For this review, take the finished solid that the model builds, in its own axes (mm). Round coordinates to 2 decimals unless told otherwise and drop trailing zeros. Write each loop counter-clockwise with the first axis right and the second up, starting at its lowest first coordinate (ties: lowest second). Pieces come first, ordered by that corner, then holes. Notation, with made-up numbers: M 15,-15.5 L 58,-15.5 A24 cw 58,15.5 Z; hole C 8.5,27 d6. An arc over 180 degrees is marked long. Use one line per item in the form item = value. Start each with the question number.
Item 1: For P1, Ø4, axis at x = 19, z = -24.5, coming from the -Y side; P2, Ø1.5, axis at x = -39, z = 24.5, coming from the -Y side, all flat-tipped, find the tip position at first contact; note any pin that passes through.
Item 2: Add section A-A (z = 24.5). State the section outline as (x, y) points, and give its area (3 significant figures).
Item 3: Add section B-B (x = -39). State the section outline as (y, z) points.
Item 4: For line 1 (X direction, y = -0.7, z = -24.5); line 2 (Z direction, x = -39, y = -0.4); line 3 (Z direction, x = 20, y = -0.2), list the stretches that pass through material, from the lowest coordinate up. Write a range as [from, to].
from build123d import *

# Parameters (mm, degrees)
SCHIZZO1_R                   = 1.25
ESTRUSIONE_ESTRUSIONE1_DEPTH = 1.3


with BuildPart() as part:
    # Schizzo1 → Estrusione-Estrusione1 (new body)
    with BuildSketch(Plane(origin=(0, 0, 0), x_dir=(1, 0, 0), z_dir=(0, 1, 0))):
        with BuildLine():
            Line((42.5, -25.5), (42.5, 25.5))
            ThreePointArc((42.5, 25.5), (41.767766953, 27.267766953), (40, 28))
            Line((40, 28), (-40, 28))
            ThreePointArc((-40, 28), (-41.767766953, 27.267766953), (-42.5, 25.5))
            Line((-42.5, 25.5), (-42.5, -25.5))
            ThreePointArc((-42.5, -25.5), (-41.767766953, -27.267766953), (-40, -28))
            Line((-40, -28), (40, -28))
            ThreePointArc((40, -28), (41.767766953, -27.267766953), (42.5, -25.5))
        make_face()
        with Locations(Location((19, 24.5, 0), (0, 0, 90))):  # turned: the seam where the file's is
            Circle(SCHIZZO1_R, mode=Mode.SUBTRACT)
        with Locations(Location((-39, 24.5, 0), (0, 0, 90))):  # turned: the seam where the file's is
            Circle(SCHIZZO1_R, mode=Mode.SUBTRACT)
        with Locations(Location((-39, -24.5, 0), (0, 0, 90))):  # turned: the seam where the file's is
            Circle(SCHIZZO1_R, mode=Mode.SUBTRACT)
        with Locations(Location((19, -24.5, 0), (0, 0, 90))):  # turned: the seam where the file's is
            Circle(SCHIZZO1_R, mode=Mode.SUBTRACT)
    extrude(amount=-ESTRUSIONE_ESTRUSIONE1_DEPTH)


solid = part.part
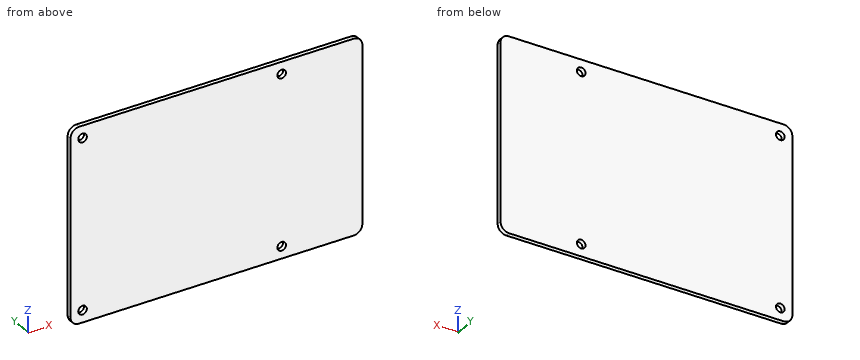
Calculated:
q1.P1 = -1.3
q1.P2 = through
q2.outline = M -42.5,-1.3 L -40.25,-1.3 L -40.25,0 L -42.5,0 Z; M -37.75,-1.3 L 17.75,-1.3 L 17.75,0 L -37.75,0 Z; M 20.25,-1.3 L 42.5,-1.3 L 42.5,0 L 20.25,0 Z
q2.area = 104 mm^2
q3.outline = M -1.3,-28 L 0,-28 L 0,-25.75 L -1.3,-25.75 Z; M -1.3,-23.25 L 0,-23.25 L 0,23.25 L -1.3,23.25 Z; M -1.3,25.75 L 0,25.75 L 0,28 L -1.3,28 Z
q4.line_1 = [-42.5, -40.25], [-37.75, 17.75], [20.25, 42.5]
q4.line_2 = [-28, -25.75], [-23.25, 23.25], [25.75, 28]
q4.line_3 = [-28, -25.25], [-23.75, 23.75], [25.25, 28]
